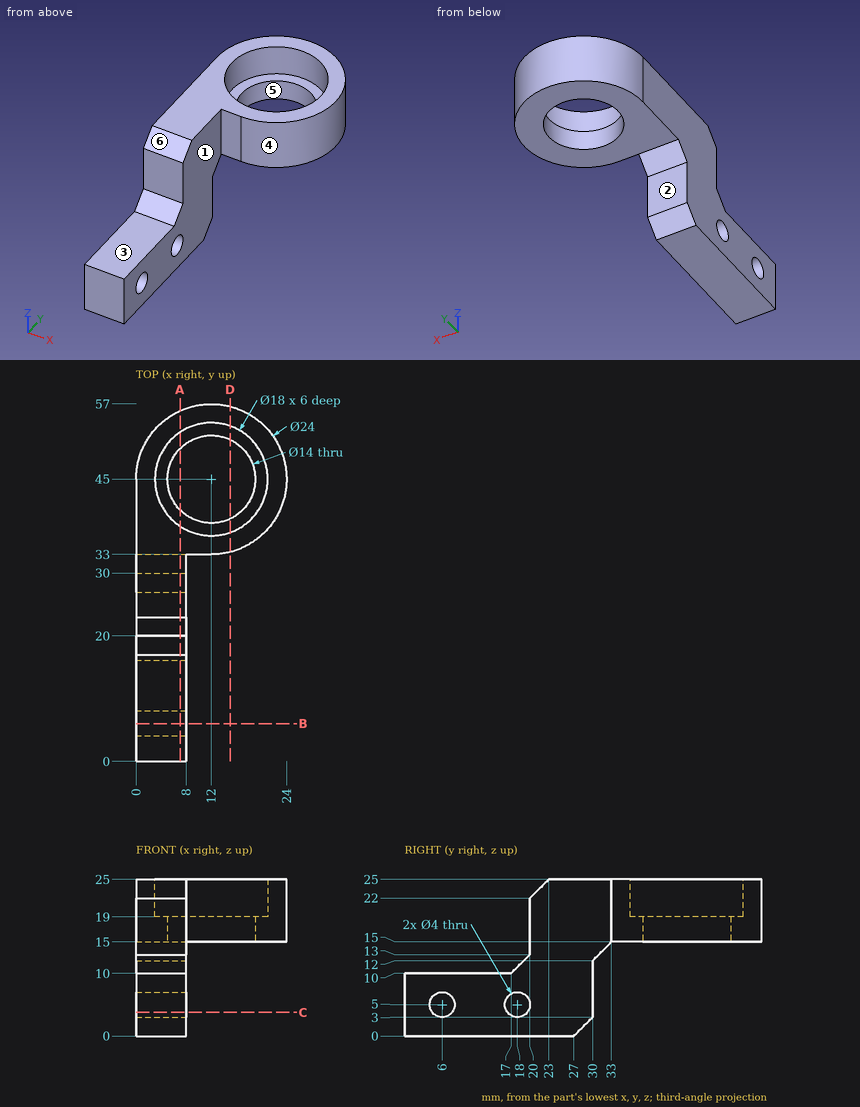
Part print with two shaded views. Sizes in mm from the minimum x, y, z corner. A direction names the side the tool comes from. Give positions to 0.01 mm unless a question says otherwise; leave off trailing zeros. Loops run counter-clockwise (first coordinate to the right, second up) from the corner with the lowest first, then second, coordinate; pieces in that order, holes last. Notation, with made-up numbers: (34.5, -20.5) -> (50.5, -20.5) arc R16 ccw to (50.5, -1.5) -> close; hole circle Ø4 at (84.25, 76). An arc over 180 degrees is marked (long way). One line per question, with ' | ' between items.
Q1. Drill centre lines: line 1 along Y through (x, z) = (4.75, 5); line 2 along Y through (x, z) = (12, 17.25); line 3 along X through (y, z) = (45, 17.6). Where is each one in solid material? Low to high. Write a range as [from, to].
Filled sheet:
line 1: y = [0, 4], [8, 16], [20, 30] | line 2: y = [33, 38], [52, 57] | line 3: x = [0, 5], [19, 24]
Q2. Drop flat-ended pins along their axis: pin 1 (4 mm diameter, centred on x = 15, y = 41.5, fed in from +Z); pin 2 (7 mm diameter, centred on x = 17, y = 41, fed in from -Z); pin 3 (4 mm diameter, centred on x = 9, y = 12, fed in from +Z); pin 4 (3 mm diameter, centred on y = 9, z = 2.5, fed in from +X). Give the stop position or say it passes through.
Filled sheet:
pin 1: passes through | pin 2: stops at z = 15 | pin 3: stops at z = 10 | pin 4: stops at x = 8
Q3. Cut at D-D, the plane x = 15. Write the cut outline in (y, z), plus the area to 3 significant figures.
Filled sheet:
outline: (33.38, 15) -> (38.68, 15) -> (38.68, 19) -> (36.51, 19) -> (36.51, 25) -> (33.38, 25) -> close; (51.32, 15) -> (56.62, 15) -> (56.62, 25) -> (53.49, 25) -> (53.49, 19) -> (51.32, 19) -> close | area: 80.0 mm²
Q4. Cut at C-C, the plane z = 3.75. Write the cut outline in (x, y), plus the area to 3 significant figures.
Filled sheet:
outline: (0, 0) -> (8, 0) -> (8, 4.44) -> (0, 4.44) -> close; (0, 7.56) -> (8, 7.56) -> (8, 16.44) -> (0, 16.44) -> close; (0, 19.56) -> (8, 19.56) -> (8, 30) -> (0, 30) -> close | area: 190 mm²
Q5. Pull direction X, two halves, no side cores. Call the marked faces 4, 5 and 6: pulls with the +X half, pulls with the -X half, needs draft (parallel to the pull), parting line crosses it, or undercut.
Filled sheet:
face 4: parting line crosses it | face 5: undercut | face 6: needs draft
Q6. Cut at B-B, the plane y = 6. Write the cut outline in (x, z), plus the area to 3 significant figures.
Filled sheet:
outline: (0, 0) -> (8, 0) -> (8, 3) -> (0, 3) -> close; (0, 7) -> (8, 7) -> (8, 10) -> (0, 10) -> close | area: 48.0 mm²
Q7. Cut at A-A, the plane x = 7. Write the cut outline in (y, z), plus the area to 3 significant figures.
Filled sheet:
outline: (0, 0) -> (27, 0) -> (30, 3) -> (30, 12) -> (33, 15) -> (40.1, 15) -> (40.1, 19) -> (37.52, 19) -> (37.52, 25) -> (23, 25) -> (20, 22) -> (20, 13) -> (17, 10) -> (0, 10) -> close; (49.9, 15) -> (55.91, 15) -> (55.91, 25) -> (52.48, 25) -> (52.48, 19) -> (49.9, 19) -> close; hole circle Ø4 at (6, 5); hole circle Ø4 at (18, 5) | area: 555 mm²
Q8. Tool access for the marked faces 1, 2 and 3: list every direction of +Z, -Z, +X, -X, +Y, -Y with a clear straight run to the whole face (end or side of a thin tool).
Filled sheet:
face 1: +Z, -Z, +X, -Y | face 2: -Z, +X, -X, +Y | face 3: +Z, +X, -X, -Y
